Check sheet for the modelled part. Datum: model origin and axes. Units: mm. A direction names the side the tool comes from. Coordinates: 2 decimals unless noted, no trailing zeros. Loops run counter-clockwise (first coordinate to the right, second up) from the corner with the lowest first, then second, coordinate; pieces in that order, holes last. Notation, with made-up numbers: (-10, 66) - (10, 66) arc R30 ccw to (10, 92) - close; hole circle Ø4 at (-32.5, 85). An arc over 180 degrees is marked (long way). Write each question's results on one line, items separated by ' | '. Start each with the question number.
1. Cross-section at A-A (x = 56). Record the cut outline in (y, z).
2. Draft check along X on faces 1 (the face through (0, 2, 41.5)), 2 (the face through (92, 1, 32)), 3 (the face through (-3, 2, 45)), 4 (the face through (4.36, 1.52, 6.4)). Enter one of: released by +X, released by -X, zero draft, split by the parting line, or undercut.
3. Gauge pin test, flat ends, axial feed: P1, Ø1.5, axis at y = 2, z = 17.5, coming from the -X side; P2, Ø8, axis at x = 44.5, z = 11.5, coming from the -Y side; P3, Ø0.9, axis at x = 49, y = 2, coming from the -Z side; P4, Ø0.9, axis at y = 1.5, z = 15.5, coming from the +X side. Record the tip position at first contact, or that the pin passes through.
4. Thickness scan on line 1 (X direction, y = 0.95, z = 48.5); line 2 (X direction, y = 1.8, z = 20.5); line 3 (Z direction, x = 28.5, y = 1.75). Record the ranges inside material, lowest first. Write a range as [from, to].
5. Tool access check on faces 5 (the face through (3.5, 2, 49)), 6 (the face through (47, 1, 0)), 7 (the face through (54, 3, 5)), 8 (the face through (-1.601, 1.521, 47.744)). Record the directions out of +Z, -Z, +X, -X, +Y, -Y that give a thin tool (end or side, any length) a straight path to the whole face; none if there is none.
6. Cross-section at B-B (z = 30.5). Record the cut outline in (x, y).
7. Cross-section at C-C (y = 1.5). Give the number of separate pieces and of enclosed holes in the cut face, and give its area (3 significant figures).
```python
from build123d import *

# Parameters (mm, degrees)
SKETCH3_R           = 2.265
BOSS_EXTRUDE2_DEPTH = 3
SKETCH4_W           = 6.5
SKETCH4_H           = 20
CUT_EXTRUDE1_DEPTH  = 3
BOSS_EXTRUDE3_DEPTH = 3
FILLET1_R           = 0.6
CUT_EXTRUDE2_DEPTH  = 3


with BuildPart() as part:
    # Sketch3 → Boss-Extrude2 (new body)
    with BuildSketch(Plane(origin=(0, 0, 0), x_dir=(1, 0, 0), z_dir=(0, 1, 0))):
        with BuildLine():
            Line((0, -4.265), (0, -58.735))
            ThreePointArc((0, -58.735), (-3.015810422, -66.015810422), (4.265, -63))
            Line((4.265, -63), (87.735, -63))
            ThreePointArc((87.735, -63), (95.015810422, -66.015810422), (92, -58.735))
            Line((92, -58.735), (92, -4.265))
            ThreePointArc((92, -4.265), (95.015810422, 3.015810422), (87.735, 0))
            Line((87.735, 0), (4.265, 0))
            ThreePointArc((4.265, 0), (-3.015810422, 3.015810422), (0, -4.265))
        make_face()
        with Locations(Location((0, 0, 0), (0, 0, 270))):
            Circle(SKETCH3_R, mode=Mode.SUBTRACT)
        with Locations(Location((92, 0, 0), (0, 0, 270))):
            Circle(SKETCH3_R, mode=Mode.SUBTRACT)
        with Locations(Location((92, -63, 0), (0, 0, 270))):
            Circle(SKETCH3_R, mode=Mode.SUBTRACT)
        with Locations(Location((0, -63, 0), (0, 0, 270))):
            Circle(SKETCH3_R, mode=Mode.SUBTRACT)
    extrude(amount=BOSS_EXTRUDE2_DEPTH)

    # Sketch4 → Cut-Extrude1 (cut)
    with BuildSketch(Plane(origin=(0, 3, 0), x_dir=(1, 0, 0), z_dir=(0, 1, 0))):
        with Locations((3.25, -31.5)):
            Rectangle(SKETCH4_W, SKETCH4_H)
    extrude(amount=-CUT_EXTRUDE1_DEPTH, mode=Mode.SUBTRACT)

    # Sketch5 → Boss-Extrude3 (add)
    with BuildSketch(Plane(origin=(0, 3, 0), x_dir=(1, 0, 0), z_dir=(0, 1, 0))):
        with BuildLine():
            Line((0, -21.5), (-2.5, -21.5))
            ThreePointArc((-2.5, -21.5), (-2.853553391, -21.353553391), (-3, -21))
            Line((-3, -21), (-3, -15.8))
            ThreePointArc((-3, -15.8), (-2.912132034, -15.587867966), (-2.7, -15.5))
            Line((-2.7, -15.5), (0, -14.9))
            Line((0, -14.9), (0, -21.5))
        make_face()
        with BuildLine():
            Line((-3, -42), (-3, -47.2))
            ThreePointArc((-3, -47.2), (-2.912132034, -47.412132034), (-2.7, -47.5))
            Line((-2.7, -47.5), (0, -48.1))
            Line((0, -48.1), (0, -41.5))
            Line((0, -41.5), (-2.5, -41.5))
            ThreePointArc((-2.5, -41.5), (-2.853553391, -41.646446609), (-3, -42))
        make_face()
    extrude(amount=-BOSS_EXTRUDE3_DEPTH)

    # Fillet1
    fillet1_edges = [part.edges().sort_by_distance(p)[0] for p in [
        (92, 1.5, 4.265),
        (92, 1.5, 58.735),
        (87.735, 1.5, 63),
        (4.265, 1.5, 63),
        (0, 1.5, 58.735),
        (0, 1.5, 4.265),
        (4.265, 1.5, 0),
        (87.735, 1.5, 0),
        (6.5, 1.5, 21.5),
        (6.5, 1.5, 41.5),
        (0, 1.5, 14.9),
        (0, 1.5, 48.1),
    ]]
    fillet(fillet1_edges, radius=FILLET1_R)

    # Sketch7 → Cut-Extrude2 (cut)
    with BuildSketch(Plane(origin=(0, 3, 0), x_dir=(1, 0, 0), z_dir=(0, 1, 0))):
        with BuildLine():
            Line((6.5, -5.5), (84, -5.5))
            ThreePointArc((84, -5.5), (86.121320344, -6.378679656), (87, -8.5))
            Line((87, -8.5), (87, -57))
            ThreePointArc((87, -57), (86.121320344, -59.121320344), (84, -60))
            Line((84, -60), (6.5, -60))
            ThreePointArc((6.5, -60), (4.378679656, -59.121320344), (3.5, -57))
            Line((3.5, -57), (3.5, -8.5))
            ThreePointArc((3.5, -8.5), (4.378679656, -6.378679656), (6.5, -5.5))
        make_face()
    extrude(amount=-CUT_EXTRUDE2_DEPTH, mode=Mode.SUBTRACT)


solid = part.part
```
Established:
1) outline: (0, 0) - (3, 0) - (3, 5.5) - (0, 5.5) - close; (0, 60) - (3, 60) - (3, 63) - (0, 63) - close
2) face 1: zero draft | face 2: released by +X | face 3: released by -X | face 4: undercut
3) P1: x = -3 | P2: through | P3: z = 0 | P4: x = 92
4) line 1: [-0.01, 3.5], [87, 92] | line 2: [-3, 3.5], [87, 92] | line 3: [0, 5.5], [60, 63]
5) face 5: +Y, -Y | face 6: -Z, +Y, -Y | face 7: +Z, -Z, +X, -X, +Y | face 8: -X, +Y, -Y
6) outline: (87, 0) - (92, 0) - (92, 3) - (87, 3) - close
7) separate pieces: 1 | enclosed holes: 4 | area: 1,330 mm^2
